Could you check a few things on this model? Use its own coordinates, in mm. Face numbers are marked on the shaded views. A direction names the side the tool comes from. Round coordinates to 2 decimals unless told otherwise and drop trailing zeros. Write each loop counter-clockwise with the first axis right and the second up, starting at its lowest first coordinate (ties: lowest second). Pieces come first, ordered by that corner, then holes. Notation, with made-up numbers: (40, -33.75) -> (65, -33.75) arc R9 cw to (65, -25.75) -> close; hole circle Ø3 at (58.25, 45). An arc over 180 degrees is marked (long way). Answer in a Markdown table with one row per item. Add a question column.
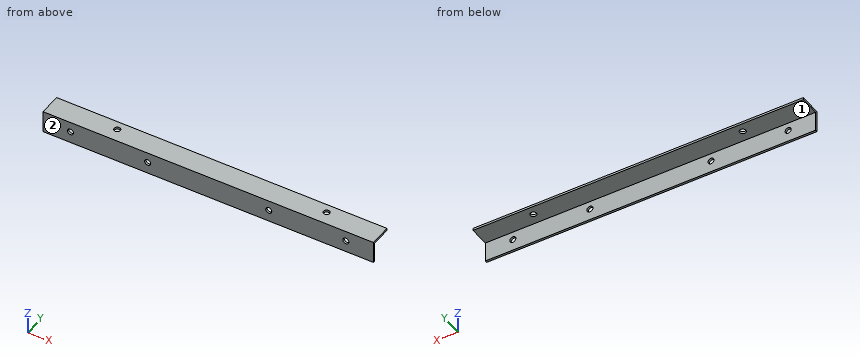
Autodesk Inventor part; units mm, degrees
ref_plane "XZ Plane" through (0, 0, 0) normal (0, 1, 0) x (-1, 0, 0)
ref_plane "XY Plane" through (0, 0, 0) normal (0, 0, 1) x (1, 0, 0)
sketch "Sketch1" plane through (0, 0, 0) normal (0, 1, 0) x (-1, 0, 0)
  line L0 (0, 0) -> (-300, 0)
  line L1 (-300, 0) -> (-300, -20)
  line L2 (-300, -20) -> (0, -20)
  line L3 (0, -20) -> (0, 0)
  dimension "d0" = 300
  dimension "d1" = 20
extrude "Extrusion1" add sketch "Sketch1" along normal blind 2
sketch "Sketch2" plane through (0, 2, 0) normal (0, 1, 0) x (1, 0, 0)
  line L0 (0, 0) -> (300, 0)
  line L1 (300, 0) -> (300, 2)
  line L2 (300, 2) -> (0, 2)
  line L3 (0, 2) -> (0, 0)
  dimension "d4" = 300
  dimension "d5" = 2
extrude "Extrusion2" add sketch "Sketch2" along normal blind 18
hole "Hole1" at (60, 11.9755, 0) direction (0, 0, -1) diameter 5.5 end through all
pattern_linear "Rectangular Pattern1" count 2 spacing 190.136 along (1, 0, 0) of "Hole1"
hole "Hole2" at (25, 2, -9.3924) direction (0, -1, 0) diameter 5.5 end through all
pattern_linear "Rectangular Pattern2" count 2 spacing 70 along (1, 0, 0) of "Hole2"
ref_plane "Work Plane1" through (150, 0, 0) normal (1, 0, 0) x (0, 1, 0)
mirror "Mirror1" about plane through (150, 0, 0) normal (1, 0, 0) of "Hole2", "Rectangular Pattern2"
properties part number "Lbarx1 small" material "Aluminum 6061"
(1) For P1, Ø4.5, axis at x = 25, z = -9.39, coming from the -Y side; P2, Ø2, axis at x = 181, z = -14, coming from the +Y side; P3, Ø5, axis at x = 234, y = 6.5, coming from the -Z side, each with a flat end and sliding along its axis, tell me the tip position at first contact or that it passes through.
(2) Suppose I cut it at B-B, the plane x = 139.5. Please give me the cut outline in (y, z).
(3) I need wall thicknesses on L1, parallel to Y at x = 60, z = -1.15; L2, parallel to Z at x = 25, y = 1.1; L3, parallel to Y at x = 187.5, z = -14. Which ranges of each line are inside material? Lowest first, please.
(4) Suppose I cut it at A-A, the plane x = 275. Please give me the cut outline in (y, z), then the cut area to 3 significant figures.
(5) On a 3-axis mill with a long thin cutter (end or side, diameter ignored), from which of +Z, -Z, +X, -X, +Y, -Y can I reach the whole of each face in a straight line? I mean the marked faces 1 and 2. Say none if no direction works.
(6) Suppose I cut it at C-C, the plane z = -15. Please give me the cut outline in (x, y), then the cut area to 3 significant figures.
Response:
| question | item | result |
|---|---|---|
| 1 | P1 | through |
| 1 | P2 | y = 2 |
| 1 | P3 | z = -2 |
| 2 | outline | (0, -20) -> (2, -20) -> (2, -2) -> (20, -2) -> (20, 0) -> (0, 0) -> close |
| 3 | L1 | 0 to 9.23, 14.73 to 20 |
| 3 | L2 | -20 to -12.14, -6.64 to 0 |
| 3 | L3 | 0 to 2 |
| 4 | outline | (0, -20) -> (2, -20) -> (2, -12.14) -> (0, -12.14) -> close; (0, -6.64) -> (2, -6.64) -> (2, -2) -> (20, -2) -> (20, 0) -> (0, 0) -> close |
| 4 | area | 65.0 mm² |
| 5 | face 1 | -Z, +X, -X, +Y |
| 5 | face 2 | +Z, -Z, +X, -X, -Y |
| 6 | outline | (0, 0) -> (300, 0) -> (300, 2) -> (0, 2) -> close |
| 6 | area | 600 mm² |
